Can you work these out from the drawing? Everything is in mm from the part's minimum corner. Round coordinates to 2 decimals unless told otherwise and drop trailing zeros. Write each loop counter-clockwise with the first axis right and the second up, starting at its lowest first coordinate (ties: lowest second). Pieces come first, ordered by that corner, then holes. Notation, with made-up numbers: (31.25, 78.5) -> (56.25, 78.5) arc R35 cw to (56.25, 110.5) -> close; hole circle Ø11 at (-14.5, 34). An arc over 180 degrees is marked (long way). Write item = value, one per line. Start each with the question number.
1) Imagine slicing it at D-D, the plane x = 180.5. Please give me the cut outline in (y, z).
2) Imagine slicing it at C-C, the plane x = 40. Please give me the cut outline in (y, z).
3) Imagine slicing it at B-B, the plane z = 55. Please give me the cut outline in (x, y).
4) I'm going to push flat-ended pins straight in: pin 1 (0.9 mm diameter, centred on y = 1, z = 57, fed in from +X); pin 2 (1.5 mm diameter, centred on y = 2, z = 1, fed in from +X); pin 3 (0.9 mm diameter, centred on x = 109, y = 1, fed in from -Z); pin 4 (6.5 mm diameter, centred on x = 10, z = 111, fed in from -Y). Where does each tip first touch, or does it pass through?
5) If I drill on line 1 (X direction, y = 2, z = 48); line 2 (Z direction, x = 291, y = 2); line 3 (Z direction, x = 10, y = 1.1), over which ranges is the centre line in solid material (lowest first)?
6) Imagine slicing it at A-A, the plane y = 0.7. State how many separate pieces and enclosed holes the cut face has, then the cut area to 3 significant figures.
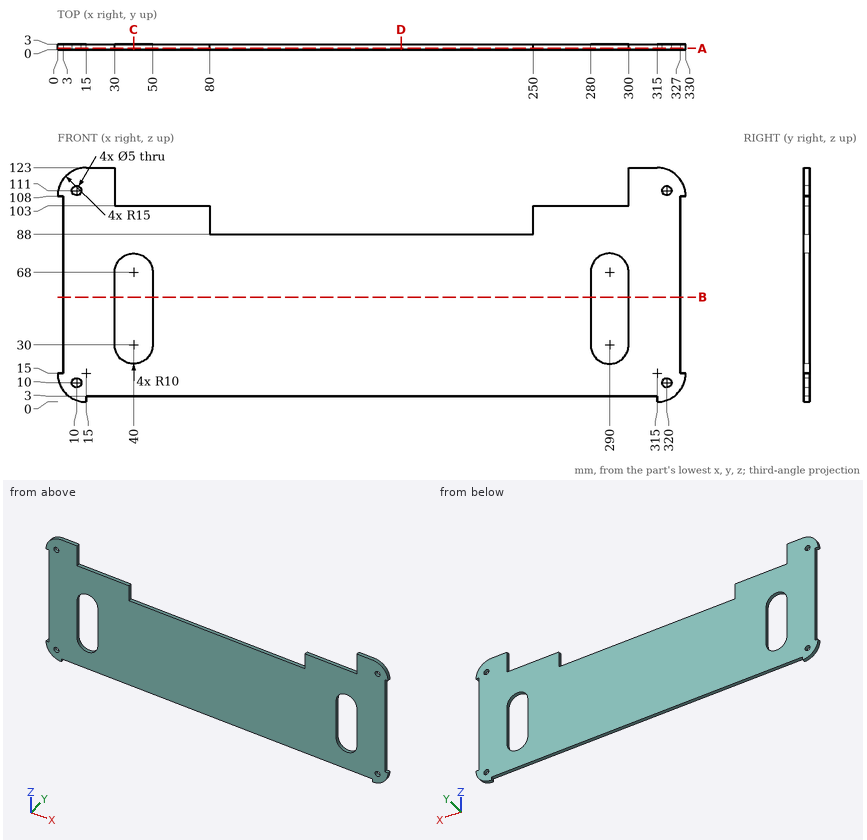
Reported:
q1.outline = (0, 3) -> (3, 3) -> (3, 88) -> (0, 88) -> close
q2.outline = (0, 3) -> (3, 3) -> (3, 20) -> (0, 20) -> close; (0, 78) -> (3, 78) -> (3, 103) -> (0, 103) -> close
q3.outline = (3, 0) -> (30, 0) -> (30, 3) -> (3, 3) -> close; (50, 0) -> (280, 0) -> (280, 3) -> (50, 3) -> close; (300, 0) -> (327, 0) -> (327, 3) -> (300, 3) -> close
q4.pin_1 = 327
q4.pin_2 = 322.03
q4.pin_3 = 3
q4.pin_4 = 0
q5.line_1 = 3 to 30, 50 to 280, 300 to 327
q5.line_2 = 3 to 20.05, 77.95 to 103
q5.line_3 = 0.86 to 7.5, 12.5 to 108.5, 113.5 to 122.14
q6.separate_pieces = 1
q6.enclosed_holes = 6
q6.area = 28,800 mm²
